Here's how the part is built. I have some questions about the finished solid (model axes, mm). A direction names the side the tool comes from. Coordinates: 2 decimals unless noted, no trailing zeros. Loops run counter-clockwise (first coordinate to the right, second up) from the corner with the lowest first, then second, coordinate; pieces in that order, holes last. Notation, with made-up numbers: (87, -20.5) -> (112, -20.5) arc R31 cw to (112, 9.5) -> close; hole circle Ø8 at (15.5, 87). An arc over 180 degrees is marked (long way). Answer as a JSON object with one key per item and string values. Group by question number.
Q1. I want a section at A-A on x = 22.5. Write out the boundary of the cut face in (y, z), then the cut area to 3 significant figures.
Q2. On a 3-axis mill with a long thin cutter (end or side, diameter ignored), from which of +Z, -Z, +X, -X, +Y, -Y can I reach the whole of each face in a straight line? I mean faces 5 (the flat face through (6, -12, 0)), 6 (the flat face through (-3.175, 0, -29)), 7 (the flat face through (3.175, 0, -29)), 8 (the flat face through (-3, -5, -23)). Say none if no direction works.
Q3. I need wall thicknesses on line 1 (Y direction, x = 11.25, z = 0.95); line 2 (Z direction, x = 4, y = -19.5); line 3 (X direction, y = 19.5, z = 1). Which ranges of each line are inside material? Lowest first, please.
Q4. I'm going to push flat-ended pins straight in: pin 1 (8.5 mm diameter, centred on x = 11.25, y = -19.49, fed in from -Z); pin 2 (13 mm diameter, centred on x = -3.5, y = -3, fed in from -Z); pin 3 (8 mm diameter, centred on y = 6, z = -27.5, fed in from +X); pin 4 (1.5 mm diameter, centred on x = 0.5, y = -8.5, fed in from -Z). Where does each tip first touch, or does it pass through?
Q5. I want a section at D-D on z = -27. Write out the boundary of the cut face in (x, y) (3 decimals), then the cut area to 3 significant figures.
Q6. I want a section at B-B on y = 0. Count the separate pieces of the cut face and the enclosed holes in it, then the cut area to 3 significant figures.
Q7. Thinking about a two-plate mould opening in Z: for faces 1 (the cylindrical face through (1.19, -5.37, -23.99)), 2 (the flat face through (-4, -4, -25)), 3 (the cylindrical face through (-7.9, -6.05, 3.49)), 4 (the flat face through (-4, 0, -26)), which applies, released by +Z, released by -Z, zero draft, split by the parting line, or undercut?
```python
from build123d import *

# Parameters (mm, degrees)
SKETCH_1_R          = 27.5
EXTRUDE_1_DEPTH     = 3
SKETCH_2_R          = 2.6
CUT_EXTRUDE_1_DEPTH = 5
SKETCH_3_R          = 9.95
EXTRUDE_2_DEPTH     = 1
SKETCH_4_R          = 8
EXTRUDE_3_DEPTH     = 13
SKETCH_5_R          = 6
EXTRUDE_4_DEPTH     = 10
SKETCH_6_R          = 5.5
EXTRUDE_5_DEPTH     = 2
SKETCH_7_R          = 5.95
EXTRUDE_6_DEPTH     = 1
FILLET_1_R          = 5
SKETCH_8_W          = 6.35
SKETCH_8_H          = 6.377891502
EXTRUDE_7_DEPTH     = 7


with BuildPart() as part:
    # 草图1 → 凸台-拉伸1 (new body)
    with BuildSketch(Plane.XY):
        Circle(SKETCH_1_R)
    extrude(amount=EXTRUDE_1_DEPTH)

    # 草图2 → 切除-拉伸1 (cut)
    with BuildSketch(Plane.XY.offset(3)):
        with Locations((22.5, 0)):
            Circle(SKETCH_2_R)
        with Locations((11.25, -19.485571585)):
            Circle(SKETCH_2_R)
        with Locations((-11.25, -19.485571585)):
            Circle(SKETCH_2_R)
        with Locations((-22.5, 0)):
            Circle(SKETCH_2_R)
        with Locations((-11.25, 19.485571585)):
            Circle(SKETCH_2_R)
        with Locations((11.25, 19.485571585)):
            Circle(SKETCH_2_R)
    extrude(amount=-CUT_EXTRUDE_1_DEPTH, mode=Mode.SUBTRACT)

    # 草图3 → 凸台-拉伸2 (add)
    with BuildSketch(Plane.XY.offset(3)):
        Circle(SKETCH_3_R)
    extrude(amount=EXTRUDE_2_DEPTH)

    # 草图4 → 凸台-拉伸3 (add)
    with BuildSketch(Plane(origin=(0, 0, 0), x_dir=(-1, 0, 0), z_dir=(0, 0, -1))):
        with Locations(Location((0, 0, 0), (0, 0, 180))):
            Circle(SKETCH_4_R)
    extrude(amount=EXTRUDE_3_DEPTH)

    # 草图5 → 凸台-拉伸4 (add)
    with BuildSketch(Plane(origin=(0, 0, -13), x_dir=(-1, 0, 0), z_dir=(0, 0, -1))):
        Circle(SKETCH_5_R)
    extrude(amount=EXTRUDE_4_DEPTH)

    # 草图6 → 凸台-拉伸5 (add)
    with BuildSketch(Plane(origin=(0, 0, -23), x_dir=(-1, 0, 0), z_dir=(0, 0, -1))):
        Circle(SKETCH_6_R)
    extrude(amount=EXTRUDE_5_DEPTH)

    # 草图7 → 凸台-拉伸6 (add)
    with BuildSketch(Plane(origin=(0, 0, -25), x_dir=(-1, 0, 0), z_dir=(0, 0, -1))):
        Circle(SKETCH_7_R)
    extrude(amount=EXTRUDE_6_DEPTH)

    # 圆角1
    fillet_1_edges = [part.edges().sort_by_distance(p)[0] for p in [
        (-8, 0, 0),
    ]]
    fillet(fillet_1_edges, radius=FILLET_1_R)

    # 草图8 → 凸台-拉伸7 (add)
    with BuildSketch(Plane(origin=(0, 0, -26), x_dir=(-1, 0, 0), z_dir=(0, 0, -1))):
        Rectangle(SKETCH_8_W, SKETCH_8_H)
        with BuildLine():
            Line((3.175, -3.188945751), (-3.175, -3.188945751))
            ThreePointArc((-3.175, -3.188945751), (0, -4.5), (3.175, -3.188945751))
        make_face()
        with BuildLine():
            ThreePointArc((3.175, 3.188945751), (0, 4.5), (-3.175, 3.188945751))
            Line((-3.175, 3.188945751), (3.175, 3.188945751))
        make_face()
    extrude(amount=EXTRUDE_7_DEPTH)


solid = part.part
```
Result set:
{
 "1": {"outline": "(-15.81, 0) -> (-2.6, 0) -> (-2.6, 3) -> (-15.81, 3) -> close; (2.6, 0) -> (15.81, 0) -> (15.81, 3) -> (2.6, 3) -> close", "area": "79.3 mm²"},
 "2": {"face 5": "-Z", "face 6": "-Z, -X, +Y, -Y", "face 7": "-Z, +X, +Y, -Y", "face 8": "none"},
 "3": {"line 1": "y = -25.09 to -22.09, -16.89 to 16.89, 22.09 to 25.09", "line 2": "z = 0 to 3", "line 3": "x = -19.39 to -13.85, -8.65 to 8.65, 13.85 to 19.39"},
 "4": {"pin 1": "stops at z = 0", "pin 2": "stops at z = -33", "pin 3": "stops at x = 5.49", "pin 4": "stops at z = -13"},
 "5": {"outline": "(-3.175, -3.189) arc R4.5 ccw to (3.175, -3.189) -> (3.175, 3.189) arc R4.5 ccw to (-3.175, 3.189) -> close", "area": "52.0 mm²"},
 "6": {"separate pieces": "3", "enclosed holes": "0", "area": "571 mm²"},
 "7": {"face 1": "undercut", "face 2": "undercut", "face 3": "zero draft", "face 4": "released by -Z"}
}
